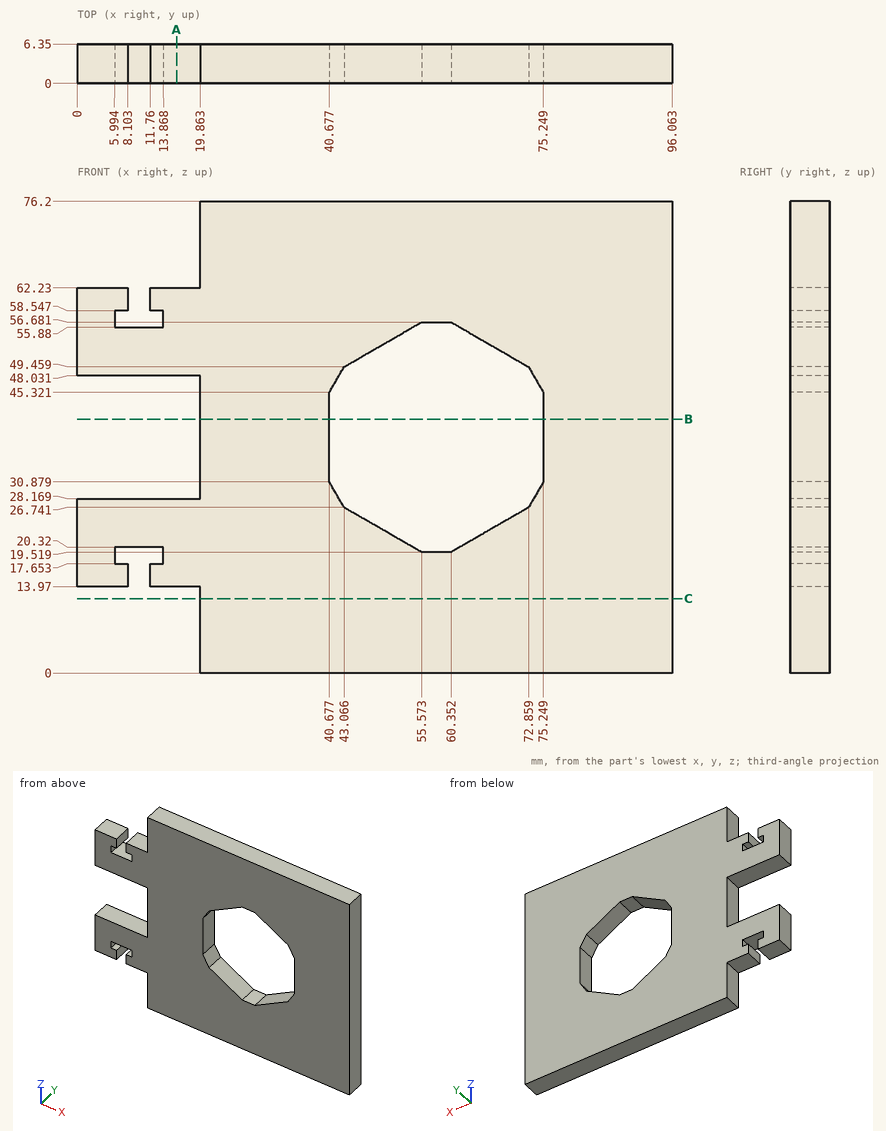
For this review, use the dimensioned drawing (mm, ordinates from the lowest corner) and the shaded views. Coordinates: 2 decimals unless noted, no trailing zeros. Write each loop counter-clockwise with the first axis right and the second up, starting at its lowest first coordinate (ties: lowest second). Pieces come first, ordered by that corner, then holes. Notation, with made-up numbers: (-20, 6.25) - (5, 6.25) arc R29 cw to (5, 33.25) - close; hole circle Ø7 at (50.25, 13). An arc over 180 degrees is marked (long way). Answer as a JSON object with one key per item and string values. Group by question number.
1. Clearance check with flat-ended pins moving along their axes: pin 1 Ø1.1 at (x, y) = (13, 4.5) entering from -Z; pin 2 Ø1.9 at (x, y) = (11, 2.5) entering from +Z. State where each tip first meets the part, or that it passes through.
2. Add section B-B (z = 41). Give the boundary of the cut face in (x, y).
3. Add section A-A (x = 16). Give the boundary of the cut face in (y, z).
4. Add section C-C (z = 12). Give the boundary of the cut face in (x, y).
5. To check wall thickness, follow probe 1 along Z at (x, y) = (56, 1.5); probe 2 along X at (y, z) = (2.75, 58.5) (1 decimal); probe 3 along Z at (x, y) = (17.5, 4). State the ranges of each line that lie inside material, in increasing order.
Findings:
{
 "1": {"pin 1": "z = 13.97", "pin 2": "z = 62.23"},
 "2": {"outline": "(19.86, 0) - (40.68, 0) - (40.68, 6.35) - (19.86, 6.35) - close; (75.25, 0) - (96.06, 0) - (96.06, 6.35) - (75.25, 6.35) - close"},
 "3": {"outline": "(0, 13.97) - (6.35, 13.97) - (6.35, 28.17) - (0, 28.17) - close; (0, 48.03) - (6.35, 48.03) - (6.35, 62.23) - (0, 62.23) - close"},
 "4": {"outline": "(19.86, 0) - (96.06, 0) - (96.06, 6.35) - (19.86, 6.35) - close"},
 "5": {"probe 1": "0 to 19.52, 56.68 to 76.2", "probe 2": "0 to 6, 13.9 to 96.1", "probe 3": "13.97 to 28.17, 48.03 to 62.23"}
}
